from build123d import *

# Parameters (mm, degrees)
F0_W          = 1
F0_H          = 10
F1_DEPTH      = 7.5
F1_DEPTH_BACK = 7.5
F2_W          = 5
F2_H          = 10
F2_H_2        = 15
F3_DEPTH      = 3
F4_R          = 1.49999
F5_R          = 4.99999


# Not quite as in the source:
# - a fillet or chamfer is up to 0.001 mm smaller than in the source, because OpenCascade refuses the exact size


with BuildPart() as f1:
    # F0 (on Right) → F1 (new body, two sides)
    with BuildSketch(Plane.YZ) as f1_sk:
        with BuildLine():
            ThreePointArc((-12, 0), (0, 12), (12, 0))
            Line((12, 0), (12, -3))
            ThreePointArc((12, -3), (13.5, -4.5), (15, -3))
            Line((15, -3), (15, 0))
            ThreePointArc((15, 0), (0, 15), (-15, 0))
            Line((-15, 0), (-15, -38))
            Line((-15, -38), (-15, -48))
            Line((-15, -48), (-12, -48))
            Line((-12, -48), (23, -48))
            Line((23, -48), (23, -60))
            Line((23, -60), (33, -60))
            Line((33, -60), (38, -60))
            Line((38, -60), (38, -55))
            Line((38, -55), (33, -55))
            Line((33, -55), (33, -48))
            Line((33, -48), (33, -38))
            Line((33, -38), (-12, -38))
            Line((-12, -38), (-12, 0))
        make_face()
        with Locations((-15.5, -43)):
            Rectangle(F0_W, F0_H)
    extrude(amount=F1_DEPTH)
    extrude(f1_sk.sketch, amount=-F1_DEPTH_BACK)

    # F2 (on face) → F3 (cut, through all)
    with BuildSketch(Plane.XZ.offset(15)):
        with Locations((0, -11)):
            Rectangle(F2_W, F2_H)
        with Locations((0, -30.5)):
            Rectangle(F2_W, F2_H_2)
    extrude(amount=-F3_DEPTH, mode=Mode.SUBTRACT)

    # F4 (radius 1.5 in the source; OpenCascade refuses exactly that, so slightly less here)
    f4_edges = [f1.edges().sort_by_distance(p)[0] for p in [
        (0, -15, -6),
        (0, -12, -6),
        (0, -15, -23),
        (0, -12, -23),
        (0, -16, -38),
    ]]
    fillet(f4_edges, radius=F4_R)

    # F5 (radius 5 in the source; OpenCascade refuses exactly that, so slightly less here)
    f5_edges = [f1.edges().sort_by_distance(p)[0] for p in [
        (5, -12, -38),
        (-5, -12, -38),
        (0, 33, -38),
        (0, 38, -60),
        (0, 23, -60),
        (0, 23, -48),
        (0, -15, 0),
        (0, -16, -48),
    ]]
    fillet(f5_edges, radius=F5_R)


solid = f1.part
Work out the finished part from the listing and answer in its coordinate system (mm). A direction names the side the tool comes from. Round coordinates to 2 decimals unless told otherwise and drop trailing zeros. Write each loop counter-clockwise with the first axis right and the second up, starting at its lowest first coordinate (ties: lowest second). Pieces come first, ordered by that corner, then holes. Notation, with made-up numbers: M 26,69.25 L 46,69.25 A28 cw 46,100.25 Z; hole C 55,-32 d9. An arc over 180 degrees is marked long. Use a Markdown table: item, result.
1) Determine the mould class of faces 1 (the face through (0, -16, -41)), 2 (the face through (0, 12, -1)), 3 (the face through (2.5, -13, -31)) for opening direction Y: pulls with the +Y half, pulls with the -Y half, needs draft (parallel to the pull), parting line crosses it, or undercut.
Taken from the geometry:
| item | result |
|---|---|
| face 1 | pulls with the -Y half |
| face 2 | undercut |
| face 3 | needs draft |
2) The part is cut by section B-B on z = -9. Give the vertices of the cut face in (x, y), plus the area to 3 significant figures.
Taken from the geometry:
| item | result |
|---|---|
| outline | M -7.5,-15 L -2.5,-15 L -2.5,-12 L -7.5,-12 Z; M 2.5,-15 L 7.5,-15 L 7.5,-12 L 2.5,-12 Z |
| area | 30.0 mm2 |
3) Which of the six approach directions +Z, -Z, +X, -X, +Y, -Y give full straight-line access (tool end or side, diameter ignored) to faces 4 (the face through (0, -12, -17)), 5 (the face through (-5, -10, -37)), 6 (the face through (0.04, -14.57, -5.55)), 7 (the face through (0, -14, -16))?
Taken from the geometry:
| item | result |
|---|---|
| face 4 | +X, -X |
| face 5 | +X, -X, +Y |
| face 6 | -Y |
| face 7 | +Y, -Y |
4) Consider line 1 (X direction, y = -12.5, z = -30); line 2 (Y direction, x = 6.5, z = -26); line 3 (Y direction, x = 0.5, z = 4). Determine where each line is inside the solid, lowest interval first. Write a range as [from, to].
Taken from the geometry:
| item | result |
|---|---|
| line 1 | x = [-7.5, -2.5], [2.5, 7.5] |
| line 2 | y = [-15, -12] |
| line 3 | y = [-14.46, -11.31], [11.31, 14.46] |
5) The part is cut by section A-A on y = 0. Give the vertices of the cut face in (x, z).
Taken from the geometry:
| item | result |
|---|---|
| outline | M -7.5,-48 L 7.5,-48 L 7.5,-38 L -7.5,-38 Z; M -7.5,12 L 7.5,12 L 7.5,15 L -7.5,15 Z |
6) Flat-ended cylindrical pins translate along their axes: pin 1 (2.5 mm diameter, centred on x = 0, y = -14, fed in from +Z); pin 2 (1 mm diameter, centred on x = -2, z = -54.5, fed in from -Y); pin 3 (1.5 mm diameter, centred on x = 0, z = -4.5, fed in from +Y). Find the tip coordinate at first contact, or state that the pin passes through.
Taken from the geometry:
| item | result |
|---|---|
| pin 1 | stops at z = 7.9 |
| pin 2 | stops at y = 23 |
| pin 3 | stops at y = 14.8 |
